Autodesk Inventor part; units mm, degrees
ref_plane "YZ Plane" through (0, 0, 0) normal (1, 0, 0) x (0, 1, 0)
ref_plane "XZ Plane" through (0, 0, 0) normal (0, 1, 0) x (-1, 0, 0)
ref_plane "XY Plane" through (0, 0, 0) normal (0, 0, 1) x (1, 0, 0)
sketch "Sketch1" plane through (0, 0, 0) normal (0, 0, 1) x (1, 0, 0)
  line L0 (0, 0) -> (5.5, 0)
  line L1 (5.5, 0) -> (5.5, 6)
  line L2 (5.5, 6) -> (4.23, 6)
  line L3 (4.23, 6) -> (4.23, 1.555)
  line L4 (0, 4.7594) -> (2, 4.7594)
  line L5 (4.23, 1.555) -> (2.96, 1.555)
  line L6 (2, 4.7594) -> (2, 4.1244)
  line L7 (2, 4.1244) -> (2.3175, 4.1244)
  arc A0 (2.3175, 5.3944) -> (2.3175, 4.1244) centre (2.7937, 4.7594) ccw
  line L8 (2.3175, 4.1244) -> (2.96, 1.555)
  line L9 (2.3175, 5.3944) -> (3.2065, 5.3944)
  arc A1 (3.2065, 5.3944) -> (3.2065, 4.1244) centre (3.9012, 4.7594) ccw
  line L10 (3.2065, 4.1244) -> (3.849, 1.555)
  line L11 (2.96, 1.555) -> (2.96, 0)
  line L12 (0, 0) -> (0, 3.2708)
  dimension "d0" = 5.5
  dimension "d1" = 6
  dimension "d2" = 1.27
  dimension "d3" = 4.445
  dimension "d4" = 2
  dimension "d5" = 1.27
  dimension "d6" = 0.635
  dimension "d7" = 0.3175
  dimension "d8" = 1.27
  dimension "d9" = 0.889
  dimension "d11" = 0.9412
revolve "Revolution1" add sketch "Sketch1" angle 360 about axis through (0, 0, 0) along (0, 1, 0) contours L11 L5 L3 L2 L1 L0 | L8 A0 L9 A1 L10 L5
properties part number "RubberMould"
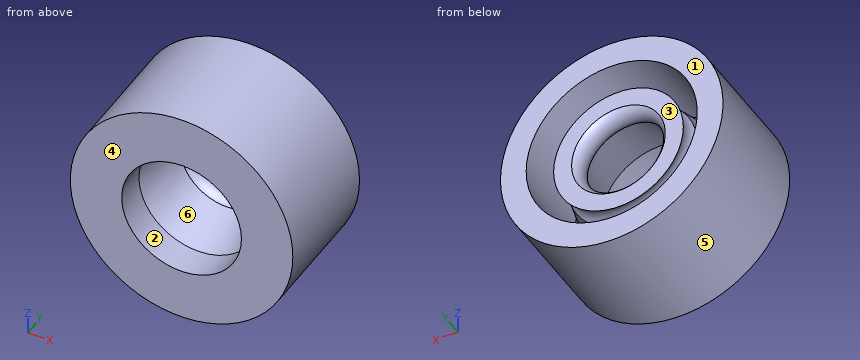
Work out the finished part from the listing and answer in its coordinate system (mm). Face numbers are marked on the shaded views. A direction names the side the tool comes from. Round coordinates to 2 decimals unless told otherwise and drop trailing zeros. Write each loop counter-clockwise with the first axis right and the second up, starting at its lowest first coordinate (ties: lowest second). Pieces come first, ordered by that corner, then holes. Notation, with made-up numbers: (84.5, 61.5) -> (95.5, 61.5) arc R21 cw to (95.5, 78.5) -> close; hole circle Ø8 at (53.25, -30.75). An arc over 180 degrees is marked (long way). Write each question's results on one line, items separated by ' | '.
Item 1: Find the intervals of material crossed by line 1 along X through (y, z) = (3.4, 0); line 2 along Z through (x, y) = (0, 0.85); line 3 along Z through (x, y) = (0, 4.8), in increasing order. Write a range as [from, to].
Result set:
line 1: [-5.5, -4.23], [-3.39, -2.5], [2.5, 3.39], [4.23, 5.5] | line 2: [-5.5, -2.96], [2.96, 5.5] | line 3: [-5.5, -4.23], [-2.96, -2], [2, 2.96], [4.23, 5.5]
Item 2: Which of the six approach directions +Z, -Z, +X, -X, +Y, -Y give full straight-line access (tool end or side, diameter ignored) to the marked faces 1, 2 and 3?
Result set:
face 1: +Z, -Z, +X, -X, +Y | face 2: -Y | face 3: +Y
Item 3: A cutting plane is placed at C-C, the plane y = 4.4. Determine the outline of the cut face in (x, z), plus the area to 3 significant figures.
Result set:
outline: circle Ø11 at (0, 0); circle Ø6.06 at (0, 0); hole circle Ø8.46 at (0, 0); hole circle Ø4.17 at (0, 0) | area: 54.0 mm^2
Item 4: The mould has two halves that part along X. Classify the marked faces 4, 5 and 6: +X half, -X half, draft (parallel to the pull), parting line (faces both ways), or undercut.
Result set:
face 4: draft | face 5: parting line | face 6: undercut
Item 5: A cutting plane is placed at D-D, the plane y = 5.2. Determine the outline of the cut face in (x, z).
Result set:
outline: circle Ø11 at (0, 0); circle Ø6.14 at (0, 0); hole circle Ø8.46 at (0, 0); hole circle Ø4.27 at (0, 0)
Item 6: A flat-ended cylindrical pin translates along its axis: P1, Ø2.5, axis at x = 1.5, z = 1, coming from the +Y side. Find the tip coordinate at first contact, or state that the pin passes through.
Result set:
P1: y = 5.39
